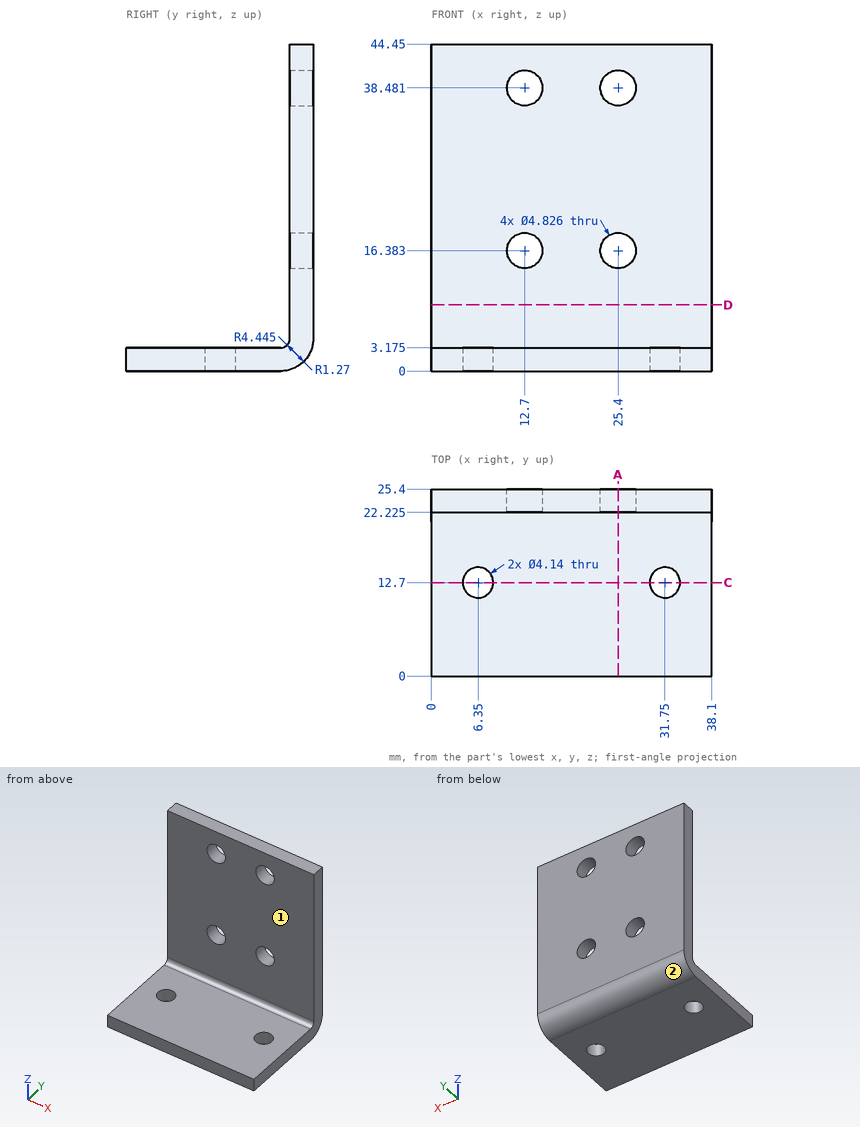
Geometry: see drawing. Coordinates: mm, zero at the bounding-box minimum. A direction names the side the tool comes from. Round coordinates to 2 decimals unless told otherwise and drop trailing zeros. Loops run counter-clockwise (first coordinate to the right, second up) from the corner with the lowest first, then second, coordinate; pieces in that order, holes last.
(1) Section query A-A (x = 25.4). Output: boundary loops of the cut face in (y, z) (3 decimals), and give its area (3 significant figures).
From the geometry:
outline: (0, 0) - (20.955, 0) arc R4.445 ccw to (25.4, 4.445) - (25.4, 13.97) - (22.225, 13.97) - (22.225, 4.445) arc R1.27 cw to (20.955, 3.175) - (0, 3.175) - close; (22.225, 18.796) - (25.4, 18.796) - (25.4, 36.068) - (22.225, 36.068) - close; (22.225, 40.894) - (25.4, 40.894) - (25.4, 44.45) - (22.225, 44.45) - close
area: 177 mm2
(2) Access query for the marked faces 1 and 2. Directions: +Z, -Z, +X, -X, +Y, -Y. A direction counts if a zero-diameter tool reaches every point of the face in a straight line with its end or side. Return the directions, or none.
From the geometry:
face 1: +Z, +X, -X, -Y
face 2: -Z, +X, -X, +Y
(3) Section query C-C (y = 12.7). Output: boundary loops of the cut face in (x, z) (1 decimal).
From the geometry:
outline: (0, 0) - (4.3, 0) - (4.3, 3.2) - (0, 3.2) - close; (8.4, 0) - (29.7, 0) - (29.7, 3.2) - (8.4, 3.2) - close; (33.8, 0) - (38.1, 0) - (38.1, 3.2) - (33.8, 3.2) - close
(4) Section query D-D (z = 9). Output: boundary loops of the cut face in (x, y) (3 decimals), and give its area (3 significant figures).
From the geometry:
outline: (0, 22.225) - (38.1, 22.225) - (38.1, 25.4) - (0, 25.4) - close
area: 121 mm2
(5) Material intervals for probe 1 along Z at (x, y) = (12.7, 23.2); probe 2 along Y at (x, z) = (33.5, 39) (3 decimals); probe 3 along Z at (x, y) = (2, 12.5) (3 decimals), sorted ascending.
From the geometry:
probe 1: z = 0.61 to 13.97, 18.8 to 36.07, 40.89 to 44.45
probe 2: y = 22.225 to 25.4
probe 3: z = 0 to 3.175
(6) Contact query for flat-ended pins moving along their axis: pin 1 Ø1 at (x, y) = (23.5, 16.5) entering from +Z (3 decimals); pin 2 Ø4.5 at (x, z) = (12.7, 16.383) entering from +Y; pin 3 Ø3 at (x, z) = (32, 15.5) entering from -Y (3 decimals). Output: stop coordinate, or through.
From the geometry:
pin 1: stops at z = 3.175
pin 2: passes through
pin 3: stops at y = 22.225
